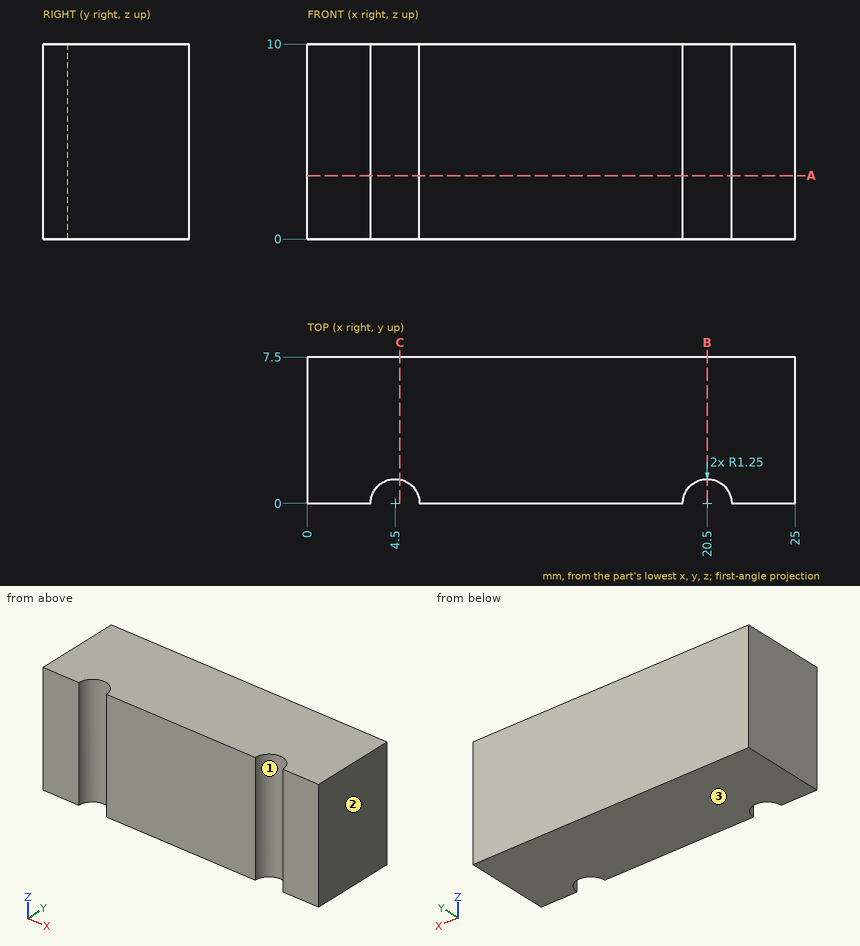
Print and shaded views of the part. All mm, measured from the part's lowest x, y and z. Coordinates: 2 decimals unless noted, no trailing zeros. Order: outer loops, then holes, each group sorted by start corner. A loop starts at its lowest first (then second) coordinate and runs counter-clockwise, first axis right, second up.
Item 1: Saw through at A-A on z = 3.25. List the corners of the cut face in (x, y), then the cut area to 3 significant figures.
Filled in:
outline: (0, 0) - (3.25, 0) arc R1.25 cw to (5.75, 0) - (19.25, 0) arc R1.25 cw to (21.75, 0) - (25, 0) - (25, 7.5) - (0, 7.5) - close
area: 183 mm2
Item 2: Drop a flat-ended pin along its axis: pin 1 Ø1 at (x, z) = (21.5, 2) entering from -Y. Give the stop position or say it passes through.
Filled in:
pin 1: stops at y = 0
Item 3: Saw through at C-C on x = 4.75. List the corners of the cut face in (y, z).
Filled in:
outline: (1.22, 0) - (7.5, 0) - (7.5, 10) - (1.22, 10) - close
Item 4: Saw through at B-B on x = 20.5. List the corners of the cut face in (y, z).
Filled in:
outline: (1.25, 0) - (7.5, 0) - (7.5, 10) - (1.25, 10) - close
Item 5: Drill centre lines: L1, parallel to X at y = 0.5, z = 9.5; L2, parallel to X at y = 0.75, z = 0.5; L3, parallel to Y at x = 4.5, z = 1.25. Where is each one in solid material? Low to high.
Filled in:
L1: x = 0 to 3.35, 5.65 to 19.35, 21.65 to 25
L2: x = 0 to 3.5, 5.5 to 19.5, 21.5 to 25
L3: y = 1.25 to 7.5
Item 6: Mould opens along X. For the marked faces 1, 2 and 3 say: released by +X, released by -X, zero draft, split by the parting line, or undercut.
Filled in:
face 1: undercut
face 2: released by +X
face 3: zero draft
